Autodesk Inventor part; units mm, degrees
ref_plane "YZ Plane" through (0, 0, 0) normal (1, 0, 0) x (0, 1, 0)
ref_plane "XZ Plane" through (0, 0, 0) normal (0, 1, 0) x (-1, 0, 0)
ref_plane "XY Plane" through (0, 0, 0) normal (0, 0, 1) x (1, 0, 0)
sketch "Sketch1" plane through (0, 0, 0) normal (0, 1, 0) x (-1, 0, 0)
  line L0 (0, 0) -> (-63.7459, 0)
  line L1 (-63.7459, 0) -> (-63.7459, -102.4121)
  line L2 (-63.7459, -102.4121) -> (0, -102.4121)
  line L3 (0, -102.4121) -> (0, 0)
  line L4 (-57.4973, -89.9149) -> (-63.7459, -89.9149)
  line L5 (-63.7459, -89.9149) -> (-63.7459, -20.7341)
  circle A0 centre (-31.873, -51.2061) radius 6.35
extrude "Extrusion1" add sketch "Sketch1" along normal blind 7 contours L3 L2 L1 L0 | A0
sketch "Sketch2" plane through (0, 7, 0) normal (0, 1, 0) x (1, 0, 0)
  line L0 (63.7459, 0) -> (63.7459, 102.4121)
  line L1 (63.7459, 19.5256) -> (58.7459, 19.5256)
  line L2 (58.7459, 19.5256) -> (58.7459, 84.196)
  line L3 (58.7459, 84.196) -> (63.7459, 84.196)
  line L4 (63.7459, 84.196) -> (63.7459, 19.5256)
  point P0 (0, 0)
  dimension "d37" = 5
extrude "Extrusion2" add sketch "Sketch2" along normal blind 40
sketch "Sketch3" plane through (0, 47, 0) normal (0, 1, 0) x (1, 0, 0)
  point P0 (0, 0)
sketch "Sketch4" plane through (0, 47, 0) normal (0, 1, 0) x (1, 0, 0)
  line L0 (63.6489, 19.5244) -> (25.7429, 19.5244)
  line L1 (25.7429, 19.5244) -> (25.7429, 84.2091)
  line L2 (25.7429, 84.2091) -> (63.6489, 84.2091)
  line L3 (63.6489, 84.2091) -> (63.6489, 19.5244)
  point P0 (0, 0)
extrude "Extrusion3" add sketch "Sketch4" along normal blind 2
hole "Hole1" at (33.3915, 49, -39.6826) direction (0, -1, 0) diameter 4.826 end up to surface
hole "Hole2" at (40.6045, 49, -39.7222) direction (0, -1, 0) diameter 4.826 depth 4.7625
hole "Hole3" at (47.4379, 49, -39.912) direction (0, -1, 0) diameter 4.826 depth 4.7625
hole "Hole4" at (31.3368, 0, -49.1509) direction (0, 1, 0) diameter 12.7 depth 7.725
Geometry check sheet. Reference: the model listing, model coordinates, mm. A direction names the side the tool comes from. Coordinates: 2 decimals unless noted, no trailing zeros. Write each loop counter-clockwise with the first axis right and the second up, starting at its lowest first coordinate (ties: lowest second). Pieces come first, ordered by that corner, then holes. Notation, with made-up numbers: M -36.75,36.25 L -6.75,36.25 A19 cw -6.75,70.25 Z; hole C 36.5,32.25 d7. An arc over 180 degrees is marked long. Use one line per item in the form item = value. Start each with the question number.
1) Go/stop test with flat-tipped pins: pin 1 Ø8 at (y, z) = (15.5, -69.5) entering from -X; pin 2 Ø2 at (x, y) = (36.5, 47.5) entering from +Z; pin 3 Ø1.6 at (x, y) = (43, 48.5) entering from -Z. Record where each tip stops, or that it passes through.
2) Section check A-A on z = -48. Enter the section's corners in (x, y).
3) Set-up check for faces 4 (the flat face through (58.746, 27, -51)), 5 (the flat face through (25.743, 48, -51)), 6 (the flat face through (45, 48, -19.524)): record each of +Z, -Z, +X, -X, +Y, -Y from which the full face is reachable in a straight line by a thin tool's end or side.
4) Section check C-C on x = 16.5. Enter the section's corners in (y, z).
5) Section check D-D on y = 36. Enter the section's corners in (x, z), and give its area (3 significant figures).
6) Release check for a two-part mould opening along Z. For faces 1 (the flat face through (44, 48, -84.209)), 2 (the flat face through (44, 47, -52)), 3 (the cylindrical face through (29.4, 3.5, -55.2)) record: pulls with the +Z half, pulls with the -Z half, needs draft (parallel to the pull), parting line crosses it, or undercut.
7) Section check B-B on z = -81.5. Enter the section's corners in (x, y), and give its area (3 significant figures).
8) Thickness scan on probe 1 along Y at (x, z) = (55, -77); probe 2 along Y at (x, z) = (25, -98); probe 3 along X at (y, z) = (37, -43.5). Record the ranges inside material, lowest first. Write a range as from..to.
Responses:
q1.pin_1 = 58.75
q1.pin_2 = -19.52
q1.pin_3 = -84.21
q2.outline = M 0,0 L 25.09,0 L 25.09,7 L 0,7 Z; M 25.74,47 L 58.75,47 L 58.75,7 L 37.58,7 L 37.58,0 L 63.75,0 L 63.75,47 L 63.65,47 L 63.65,49 L 25.74,49 Z
q3.face_4 = +Z, -Z, -X
q3.face_5 = +Z, -Z, -X, +Y
q3.face_6 = +Z, +X, -X, +Y
q4.outline = M 0,-102.41 L 7,-102.41 L 7,0 L 0,0 Z
q5.outline = M 58.75,-84.2 L 63.75,-84.2 L 63.75,-19.53 L 58.75,-19.53 Z
q5.area = 323 mm2
q6.face_1 = pulls with the -Z half
q6.face_2 = needs draft
q6.face_3 = undercut
q7.outline = M 0,0 L 63.75,0 L 63.75,47 L 63.65,47 L 63.65,49 L 25.74,49 L 25.74,47 L 58.75,47 L 58.75,7 L 0,7 Z
q7.area = 722 mm2
q8.probe_1 = 0..7, 47..49
q8.probe_2 = 0..7
q8.probe_3 = 58.75..63.75
